Input: part model. Units: mm. Frame: model coordinates. A direction names the side the tool comes from. Round coordinates to 2 decimals unless told otherwise and drop trailing zeros. Order: outer loops, then holes, each group sorted by start corner. A loop starts at its lowest first (then second) coordinate and runs counter-clockwise, first axis right, second up. Notation, with made-up numbers: (-13, 12.25) -> (29, 12.25) arc R15 ccw to (29, 23.25) -> close; hole circle Ø4 at (-40, 64.5). An arc over 180 degrees is marked (long way). Use a Markdown table: item, result.
Autodesk Inventor part; units mm, degrees
ref_plane "YZ Plane" through (0, 0, 0) normal (1, 0, 0) x (0, 1, 0)
ref_plane "XZ Plane" through (0, 0, 0) normal (0, 1, 0) x (-1, 0, 0)
ref_plane "XY Plane" through (0, 0, 0) normal (0, 0, 1) x (1, 0, 0)
sketch "Skizze1" plane through (0, 0, 0) normal (0, 1, 0) x (-1, 0, 0)
  line L0 (-44.3, 91.3) -> (44.3, 91.3)
  line L1 (44.3, 91.3) -> (44.3, -91.3)
  line L2 (44.3, -91.3) -> (-44.3, -91.3)
  line L3 (-44.3, -91.3) -> (-44.3, 91.3)
  line L4 (-44.3, 91.3) -> (44.3, -91.3) construction
  line L5 (44.3, 91.3) -> (-44.3, -91.3) construction
  point P0 (0, 0)
  dimension "d0" = 88.6
  dimension "d1" = 182.6
extrude "Extrusion1" add sketch "Skizze1" along normal blind 3
sketch "Skizze2" plane through (0, 0, 0) normal (0, -1, 0) x (1, 0, 0)
  line L0 (-44.3, -91.3) -> (44.3, -91.3)
  line L1 (0, -91.3) -> (0, 91.3)
  line L2 (44.3, 91.3) -> (-44.3, 91.3)
  line L3 (-24.5, -61.3) -> (24.5, -61.3)
  line L4 (24.5, -61.3) -> (24.5, -3.3)
  line L5 (24.5, -3.3) -> (-24.5, -3.3)
  line L6 (-24.5, -3.3) -> (-24.5, -61.3)
  line L7 (-24.5, -61.3) -> (24.5, -3.3) construction
  line L8 (24.5, -61.3) -> (-24.5, -3.3) construction
  point P0 (0, 0)
  point P1 (0, -32.3)
  dimension "d5" = 49
  dimension "d6" = 58
  dimension "d7" = 30
hole "Bohrung1" at (-24.5, 0, -61.3) at (24.5, 0, -61.3) at (24.5, 0, -3.3) at (-24.5, 0, -3.3) direction (0, 1, 0) diameter 3 depth 2.5
sketch "Skizze3" plane through (0, 0, 0) normal (0, -1, 0) x (1, 0, 0)
  line L0 (32.5, 15.0873) -> (-32.5, 15.0873)
  line L1 (-37.5, 20.0873) -> (-37.5, 20.0873)
  line L2 (-32.5, 25.0873) -> (32.5, 25.0873)
  line L3 (37.5, 20.0873) -> (37.5, 20.0873)
  line L4 (37.5, 15.0873) -> (-37.5, 25.0873) construction
  line L5 (-37.5, 15.0873) -> (37.5, 25.0873) construction
  arc A0 (-37.5, 20.0873) -> (-32.5, 15.0873) centre (-32.5, 20.0873) ccw
  arc A1 (-32.5, 25.0873) -> (-37.5, 20.0873) centre (-32.5, 20.0873) ccw
  arc A2 (32.5, 15.0873) -> (37.5, 20.0873) centre (32.5, 20.0873) ccw
  arc A3 (37.5, 20.0873) -> (32.5, 25.0873) centre (32.5, 20.0873) ccw
  point P0 (0, 0)
  point P1 (0, 20.0873)
  dimension "d15" = 75
  dimension "d16" = 10
  dimension "d18" = 5
  dimension "d19" = 5
  dimension "d20" = 5
extrude "Extrusion2" cut sketch "Skizze3" against normal blind 10
pattern_linear "Rechteckige Anordnung1" count 5 spacing 15 along (0, 0, 1) of "Extrusion2"
hole "Bohrung2" at (-39.9, 0, -87.9) direction (0, 1, 0) diameter 3 depth 8 tip angle 118
mirror "Spiegeln1" about plane through (0, 0, 0) normal (1, 0, 0) of "Bohrung2"
mirror "Spiegeln2" about plane through (0, 0, 0) normal (0, 0, 1) of "Bohrung2", "Spiegeln1"
hole "Bohrung3" at (-0.3, 0, -81.3) direction (0, 1, 0) diameter 11.8 depth 8 tip angle 118
properties part number "RaspberryBox_Backplate"
1) Contact query for a flat-ended pin moving along its axis: P1, Ø1.8, axis at x = 24.5, z = -61.3, coming from the -Y side. Output: stop coordinate, or through.
Answer key:
| item | result |
|---|---|
| P1 | stops at y = 2.5 |
2) Set-up query: faces 3 (the face through (37.5, 1.5, 50)), 4 (the face through (1, 0, -19)). Return all of +Z, -Z, +X, -X, +Y, -Y with unobstructed straight access to the full face (end or side cutting, diameter ignored); none if empty.
Answer key:
| item | result |
|---|---|
| face 3 | +Y, -Y |
| face 4 | +Z, -Z, +X, -X, -Y |
3) Cut plane B-B on y = 1.9. State how many separate pieces and enclosed holes the cut face has, and give its area (3 significant figures).
Answer key:
| item | result |
|---|---|
| separate pieces | 1 |
| enclosed holes | 14 |
| area | 12,400 mm^2 |
4) Cut plane C-C on z = 52. Return loops of the section in (x, y), and give its area (3 significant figures).
Answer key:
| item | result |
|---|---|
| outline | (-44.3, 0) -> (-37.12, 0) -> (-37.12, 3) -> (-44.3, 3) -> close; (37.12, 0) -> (44.3, 0) -> (44.3, 3) -> (37.12, 3) -> close |
| area | 43.1 mm^2 |
5) Ray query, probe 1 along X at (y, z) = (0.75, -3.3); probe 2 along X at (y, z) = (2.2, -87.9); probe 3 along Z at (x, y) = (18.5, 0.4). Return the intervals inside material, ascending.
Answer key:
| item | result |
|---|---|
| probe 1 | x = -44.3 to -26, -23 to 23, 26 to 44.3 |
| probe 2 | x = -44.3 to -41.4, -38.4 to 38.4, 41.4 to 44.3 |
| probe 3 | z = -91.3 to 15.09, 25.09 to 30.09, 40.09 to 45.09, 55.09 to 60.09, 70.09 to 75.09, 85.09 to 91.3 |
6) Draft query along Z for faces 1 (the face through (1.96, 1.52, -86.75)), 2 (the face through (1, 3, -19)). Return one class per face: released by +Z, released by -Z, zero draft, split by the parting line, or undercut.
Answer key:
| item | result |
|---|---|
| face 1 | undercut |
| face 2 | zero draft |
7) Cut plane A-A on x = 10. Return loops of the section in (y, z).
Answer key:
| item | result |
|---|---|
| outline | (0, -91.3) -> (3, -91.3) -> (3, 15.09) -> (0, 15.09) -> close; (0, 25.09) -> (3, 25.09) -> (3, 30.09) -> (0, 30.09) -> close; (0, 40.09) -> (3, 40.09) -> (3, 45.09) -> (0, 45.09) -> close; (0, 55.09) -> (3, 55.09) -> (3, 60.09) -> (0, 60.09) -> close; (0, 70.09) -> (3, 70.09) -> (3, 75.09) -> (0, 75.09) -> close; (0, 85.09) -> (3, 85.09) -> (3, 91.3) -> (0, 91.3) -> close |
8) Cut plane D-D on x = -3. Return loops of the section in (y, z).
Answer key:
| item | result |
|---|---|
| outline | (0, -91.3) -> (3, -91.3) -> (3, -86.55) -> (0, -86.55) -> close; (0, -76.05) -> (3, -76.05) -> (3, 15.09) -> (0, 15.09) -> close; (0, 25.09) -> (3, 25.09) -> (3, 30.09) -> (0, 30.09) -> close; (0, 40.09) -> (3, 40.09) -> (3, 45.09) -> (0, 45.09) -> close; (0, 55.09) -> (3, 55.09) -> (3, 60.09) -> (0, 60.09) -> close; (0, 70.09) -> (3, 70.09) -> (3, 75.09) -> (0, 75.09) -> close; (0, 85.09) -> (3, 85.09) -> (3, 91.3) -> (0, 91.3) -> close |
